Solid Edge part; units mm, degrees
sketch "Sketch1" plane through (0, 0, 0) normal (0, -1, 0) x (1, 0, 0)
  line L0 (0, 20.7) -> (4.505, 20.7)
  line L1 (4.505, 20.7) -> (4.505, 17.25)
  line L2 (4.505, 17.25) -> (2.1, 17.25)
  line L3 (2.1, 17.25) -> (2.1, 16.85)
  line L4 (2.1, 16.85) -> (2.5, 16.85)
  line L5 (2.5, 16.85) -> (2.5, 7.25)
  line L6 (2.5, 7.25) -> (2, 7.25)
  line L7 (2, 7.25) -> (2, 0)
  line L8 (2, 0) -> (0, 0)
  dimension "D1" = 4.505
  dimension "D2" = 2.1
  dimension "D3" = 2
  dimension "D4" = 2.5
  dimension "D5" = 2
revolve "RevolvedProtrusion1" add sketch "Sketch1" angle 360 about axis through (0, 0, 0) along (0, 0, 1)
chamfer "Chamfer1" distance 0.3 angle 45 3 edges at (-2.5, 0, 16.85) (-4.505, 0, 20.7) (-2, 0, 0)
fillet "Round_1" radius 0.2 4 edges at (-4.505, 0, 17.25) (-2.1, 0, 17.25) (-2.5, 0, 7.25) (-2.5, 0, 16.55)
sketch "Sketch2" plane through (0, 0, 20.7) normal (0, 0, 1) x (1, 0, 0)
  line L0 (1.5, 0.866) -> (0, 1.7321)
  line L1 (0, 1.7321) -> (-1.5, 0.866)
  line L2 (-1.5, 0.866) -> (-1.5, -0.866)
  line L3 (-1.5, -0.866) -> (0, -1.7321)
  line L4 (0, -1.7321) -> (1.5, -0.866)
  line L5 (1.5, -0.866) -> (1.5, 0.866)
extrude "ExtrudedCutout_1" cut sketch "Sketch2" against normal blind 2.4
Geometry check sheet. Reference: the model listing, model coordinates, mm. A direction names the side the tool comes from. Round coordinates to 2 decimals unless told otherwise and drop trailing zeros. Loops run counter-clockwise (first coordinate to the right, second up) from the corner with the lowest first, then second, coordinate; pieces in that order, holes last. Notation, with made-up numbers: (23, -13.5) - (42, -13.5) arc R19 cw to (42, 1.5) - close; hole circle Ø2 at (2.25, 42.25). An arc over 180 degrees is marked (long way). One line per question, with ' | ' between items. Start each with the question number.
1. Draft check along X on faces 4 (the face through (-0.74, 1.305, 19.517)), 5 (the face through (4.3, -1.35, 18.9)), 6 (the face through (2, -2, 17.25)). Enter one of: released by +X, released by -X, zero draft, split by the parting line, or undercut.
2. Tool access check on faces 1 (the face through (0, 0, 0)), 2 (the face through (-1.5, 0, 20)), 3 (the face through (-0.54, 2.44, 11.9)). Record the directions out of +Z, -Z, +X, -X, +Y, -Y that give a thin tool (end or side, any length) a straight path to the whole face; none if there is none.
3. Depth check by flat-ended pin: pin 1 (4 mm diameter, centred on y = -1.5, z = 3, fed in from -X); pin 2 (4 mm diameter, centred on y = 2, z = 6, fed in from +X); pin 3 (5 mm diameter, centred on x = 1.5, z = 15, fed in from +Y). Enter the tip coordinate at first touch or a pass-through.
4. Cross-section at A-A on z = 18.75. Record the cut outline in (x, y) (3 decimals), then the cut area to 3 significant figures.
5. Cross-section at B-B on z = 6.5. Record the cut outline in (x, y).
6. Cross-section at C-C on z = 9.75. Record the cut outline in (x, y), then the cut area to 3 significant figures.
7. Scan lines: line 1 (X direction, y = 2, z = 15.25); line 2 (Z direction, x = -1.25, y = -0.75); line 3 (Z direction, x = -0.25, y = 3). Record each from-to range of solid material in increasing order. Write a range as [from, to].
Taken from the geometry:
1) face 4: undercut | face 5: split by the parting line | face 6: zero draft
2) face 1: -Z, +X, -X, +Y, -Y | face 2: +Z | face 3: -Z
3) pin 1: x = -2 | pin 2: x = 2.43 | pin 3: y = 4.43
4) outline: circle Ø9.01 at (0, 0); hole (-1.5, -0.866) - (0, -1.732) - (1.5, -0.866) - (1.5, 0.866) - (0, 1.732) - (-1.5, 0.866) - close | area: 56.0 mm²
5) outline: circle Ø4 at (0, 0)
6) outline: circle Ø5 at (0, 0) | area: 19.6 mm²
7) line 1: [-1.5, 1.5] | line 2: [0, 18.3] | line 3: [17.25, 20.7]
